Work out the finished part from the listing and answer in its coordinate system (mm). Face numbers are marked on the shaded views. A direction names the side the tool comes from. Coordinates: 2 decimals unless noted, no trailing zeros. Order: outer loops, then holes, each group sorted by start corner. A loop starts at its lowest first (then second) coordinate and runs counter-clockwise, first axis right, second up. Notation, with made-up numbers: (8.5, 36.5) - (16.5, 36.5) arc R31 ccw to (16.5, 60.5) - close; hole circle Ø7 at (62.5, 24.25). An arc over 180 degrees is marked (long way). Use CSV: the item, a comma, the result in double quotes. Start each with the question number.
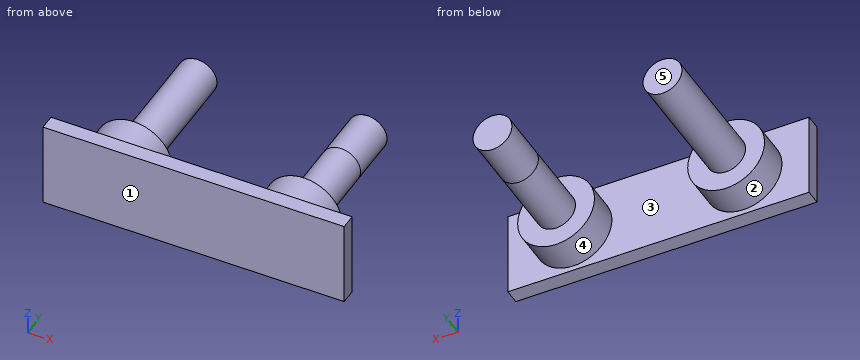
from build123d import *

# Parameters (mm, degrees)
F0_W     = 29.399694
F0_H     = 8.449018
F0_R     = 3.75
F0_R_2   = 1.9
F1_DEPTH = 11.78
F2_DEPTH = 10.28
F3_DEPTH = 7
F4_DEPTH = 5


with BuildPart() as f1:
    # F0 (on Front) → F1 (new body)
    with BuildSketch(Plane.XZ):
        Rectangle(F0_W, F0_H)
        with Locations((-8.3, 0)):
            Circle(F0_R, mode=Mode.SUBTRACT)
        with Locations((8.3, 0)):
            Circle(F0_R, mode=Mode.SUBTRACT)
        with Locations((-8.3, 0)):
            Circle(F0_R)
        with Locations((-8.3, 0)):
            Circle(F0_R_2, mode=Mode.SUBTRACT)
        with Locations((-8.3, 0)):
            Circle(F0_R_2)
        with Locations((8.3, 0)):
            Circle(F0_R)
        with Locations((8.3, 0)):
            Circle(F0_R_2, mode=Mode.SUBTRACT)
        with Locations((8.3, 0)):
            Circle(F0_R_2)
    extrude(amount=F1_DEPTH)

    # F0 (on Front) → F2 (cut)
    with BuildSketch(Plane.XZ):
        Rectangle(F0_W, F0_H)
        with Locations((-8.3, 0)):
            Circle(F0_R, mode=Mode.SUBTRACT)
        with Locations((8.3, 0)):
            Circle(F0_R, mode=Mode.SUBTRACT)
    extrude(amount=F2_DEPTH, mode=Mode.SUBTRACT)

    # F0 (on Front) → F3 (cut)
    with BuildSketch(Plane.XZ):
        with Locations((-8.3, 0)):
            Circle(F0_R)
        with Locations((-8.3, 0)):
            Circle(F0_R_2, mode=Mode.SUBTRACT)
        with Locations((8.3, 0)):
            Circle(F0_R)
        with Locations((8.3, 0)):
            Circle(F0_R_2, mode=Mode.SUBTRACT)
    extrude(amount=F3_DEPTH, mode=Mode.SUBTRACT)

    # F0 (on Front) → F4 (join)
    with BuildSketch(Plane.XZ):
        with Locations((-8.3, 0)):
            Circle(F0_R_2)
        with Locations((8.3, 0)):
            Circle(F0_R_2)
    extrude(amount=-F4_DEPTH)


solid = f1.part
1) For a pull along X with two mould halves and no side action, classify the marked faces 3, 4 and 5 as +X half, -X half, draft (parallel to the pull), parting line (faces both ways), or undercut.
2) The part is cut by section D-D on z = 2.25. Determine the outline of the cut face in (x, y), plus the area to 3 significant figures.
3) Straight lines are drawn through the part: line 1 (Y direction, x = 12.75, z = -0.75); line 2 (Y direction, x = -11, z = -1.5); line 3 (X direction, y = -3, z = -0.25). For each, find the intervals that lie inside material, in ascending order. Write a range as [from, to].
4) For the marked faces 1 and 2, determine the directions among +Z, -Z, +X, -X, +Y, -Y from which every point of the face is accessible in a straight line to the end or side of a thin tool.
5) Flat-ended cylindrical pins translate along their axes: P1, Ø5, axis at y = 0, z = -1, coming from the +X side; P2, Ø2.5, axis at x = 2, z = 1.5, coming from the +Y side. Find the tip coordinate at first contact, or state that the pin passes through.
6) The part is cut by section A-A on y = -3.5. Determine the outline of the cut face in (x, z).
7) The part is cut by section B-B on z = 0. Determine the outline of the cut face in (x, y).
8) The part is cut by section C-C on x = -8.3. Determine the outline of the cut face in (y, z), plus the area to 3 significant figures.
Answer key:
1,face 3,"undercut"
1,face 4,"undercut"
1,face 5,"draft"
2,outline,"(-14.7, -11.78) - (14.7, -11.78) - (14.7, -10.28) - (11.3, -10.28) - (11.3, -7) - (5.3, -7) - (5.3, -10.28) - (-5.3, -10.28) - (-5.3, -7) - (-11.3, -7) - (-11.3, -10.28) - (-14.7, -10.28) - close"
2,area,"83.5 mm^2"
3,line 1,"[-11.78, -10.28]"
3,line 2,"[-11.78, -7]"
3,line 3,"[-10.18, -6.42], [6.42, 10.18]"
4,face 1,"+Z, -Z, +X, -X, -Y"
4,face 2,"+Y"
5,P1,"x = 10.2"
5,P2,"y = -10.28"
6,outline,"circle Ø3.8 at (-8.3, 0); circle Ø3.8 at (8.3, 0)"
7,outline,"(-14.7, -11.78) - (14.7, -11.78) - (14.7, -10.28) - (12.05, -10.28) - (12.05, -7) - (10.2, -7) - (10.2, 5) - (6.4, 5) - (6.4, -7) - (4.55, -7) - (4.55, -10.28) - (-4.55, -10.28) - (-4.55, -7) - (-6.4, -7) - (-6.4, 5) - (-10.2, 5) - (-10.2, -7) - (-12.05, -7) - (-12.05, -10.28) - (-14.7, -10.28) - close"
8,outline,"(-11.78, -4.22) - (-10.28, -4.22) - (-10.28, -3.75) - (-7, -3.75) - (-7, -1.9) - (5, -1.9) - (5, 1.9) - (-7, 1.9) - (-7, 3.75) - (-10.28, 3.75) - (-10.28, 4.22) - (-11.78, 4.22) - close"
8,area,"82.9 mm^2"
